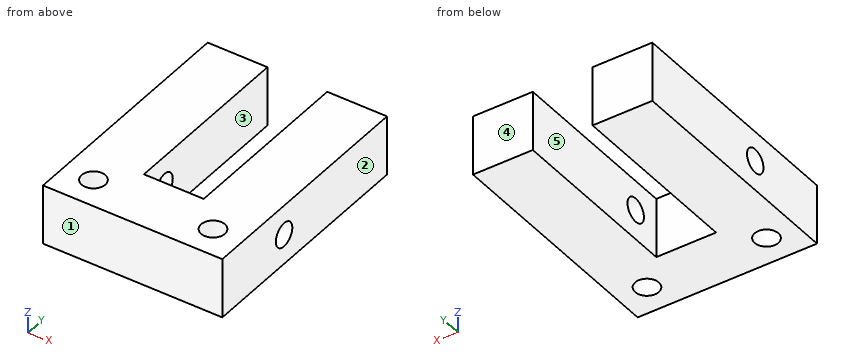
from build123d import *

# Parameters (mm, degrees)
SKETCH1_W        = 19.05
SKETCH1_H        = 25.4
MAIN_BLOCK_DEPTH = 6.35
SKETCH2_W        = 6.35
SKETCH2_H        = 19.05
U_CUT_DEPTH      = 12.7
SKETCH3_R        = 1.25603
BOLT_HOLES_DEPTH = 12.7
SKETCH4_R        = 1.27
PIN_HOLE_DEPTH   = 20.05


with BuildPart() as part:
    # Sketch1 → Main block (new body)
    with BuildSketch(Plane.XY):
        with Locations((9.525, 12.7)):
            Rectangle(SKETCH1_W, SKETCH1_H)
    extrude(amount=MAIN_BLOCK_DEPTH)

    # Sketch2 → U-cut (cut)
    with BuildSketch(Plane.XY.offset(6.35)):
        with Locations((9.525, 15.875)):
            Rectangle(SKETCH2_W, SKETCH2_H)
    extrude(amount=-U_CUT_DEPTH, mode=Mode.SUBTRACT)

    # Sketch3 → Bolt holes (cut)
    with BuildSketch(Plane.XY.offset(6.35)):
        with Locations((3.175, 3.175)):
            Circle(SKETCH3_R)
        with Locations((15.875, 3.175)):
            Circle(SKETCH3_R)
    extrude(amount=-BOLT_HOLES_DEPTH, mode=Mode.SUBTRACT)

    # Sketch4 → Pin hole (cut, through all)
    with BuildSketch(Plane.ZY):
        with Locations((3.175, 9.525)):
            Circle(SKETCH4_R)
    extrude(amount=-PIN_HOLE_DEPTH, mode=Mode.SUBTRACT)


solid = part.part
Design review of the part built by this model. Coordinates are the model's own, in mm. Face numbers are marked on the shaded views. A direction names the side the tool comes from. Round coordinates to 2 decimals unless told otherwise and drop trailing zeros. Loops run counter-clockwise (first coordinate to the right, second up) from the corner with the lowest first, then second, coordinate; pieces in that order, holes last. Notation, with made-up numbers: (39, -34.75) - (67, -34.75) arc R30 cw to (67, -10.75) - close; hole circle Ø11 at (21.5, 43). An arc over 180 degrees is marked (long way). One line per item, written item: value. Start each with the question number.
1) Consider section B-B on x = 15.75. Give the boundary of the cut face in (y, z) (3 decimals), then the cut area to 3 significant figures.
2) Draft analysis for pull direction X (two halves, no side actions). For the marked faces 1, 2 and 3, state which applies: +X half, -X half, draft (parallel to the pull), parting line (faces both ways), or undercut.
3) To check wall thickness, follow L1, parallel to X at y = 22, z = 5.75; L2, parallel to X at y = 3.75, z = 5.75; L3, parallel to Y at x = 17, z = 3. State the ranges of each line that lie inside material, in increasing order. Write a range as from..to.
4) Insertion check: pin 1 Ø3 at (x, z) = (9, 2.5) entering from +Y. The pin has a flat end and moves straight along its axis. Give the tip position at first contact, or say it passes through.
5) Consider section D-D on z = 4. Give the boundary of the cut face in (x, y) (3 decimals), then the cut area to 3 significant figures.
6) For the marked faces 4 and 5, list the 3-axis set-ups (+Z, -Z, +X, -X, +Y, -Y) from which the entire face can be reached by the end or side of a thin tool; tool diameter is ignored.
7) Consider section C-C on z = 1.5. Give the boundary of the cut face in (x, y) (3 decimals), then the cut area to 3 significant figures.
8) Consider section A-A on y = 22. Give the boundary of the cut face in (x, z), then the cut area to 3 significant figures.
Reported:
1. outline: (0, 0) - (1.925, 0) - (1.925, 6.35) - (0, 6.35) - close; (4.425, 0) - (25.4, 0) - (25.4, 6.35) - (4.425, 6.35) - close; hole circle Ø2.54 at (9.525, 3.175)
1. area: 140 mm^2
2. face 1: draft
2. face 2: +X half
2. face 3: undercut
3. L1: x = 0..6.35, 12.7..19.05
3. L2: x = 0..2.06, 4.29..14.76, 16.99..19.05
3. L3: y = 0..2.62, 3.73..8.27, 10.78..25.4
4. pin 1: stops at y = 6.35
5. outline: (0, 0) - (19.05, 0) - (19.05, 8.559) - (12.7, 8.559) - (12.7, 6.35) - (6.35, 6.35) - (6.35, 8.559) - (0, 8.559) - close; (0, 10.491) - (6.35, 10.491) - (6.35, 25.4) - (0, 25.4) - close; (12.7, 10.491) - (19.05, 10.491) - (19.05, 25.4) - (12.7, 25.4) - close; hole circle Ø2.512 at (3.175, 3.175); hole circle Ø2.512 at (15.875, 3.175)
5. area: 328 mm^2
6. face 4: +Z, -Z, +X, -X, +Y
6. face 5: +Z, -Z, +Y
7. outline: (0, 0) - (19.05, 0) - (19.05, 25.4) - (12.7, 25.4) - (12.7, 6.35) - (6.35, 6.35) - (6.35, 25.4) - (0, 25.4) - close; hole circle Ø2.512 at (3.175, 3.175); hole circle Ø2.512 at (15.875, 3.175)
7. area: 353 mm^2
8. outline: (0, 0) - (6.35, 0) - (6.35, 6.35) - (0, 6.35) - close; (12.7, 0) - (19.05, 0) - (19.05, 6.35) - (12.7, 6.35) - close
8. area: 80.6 mm^2
